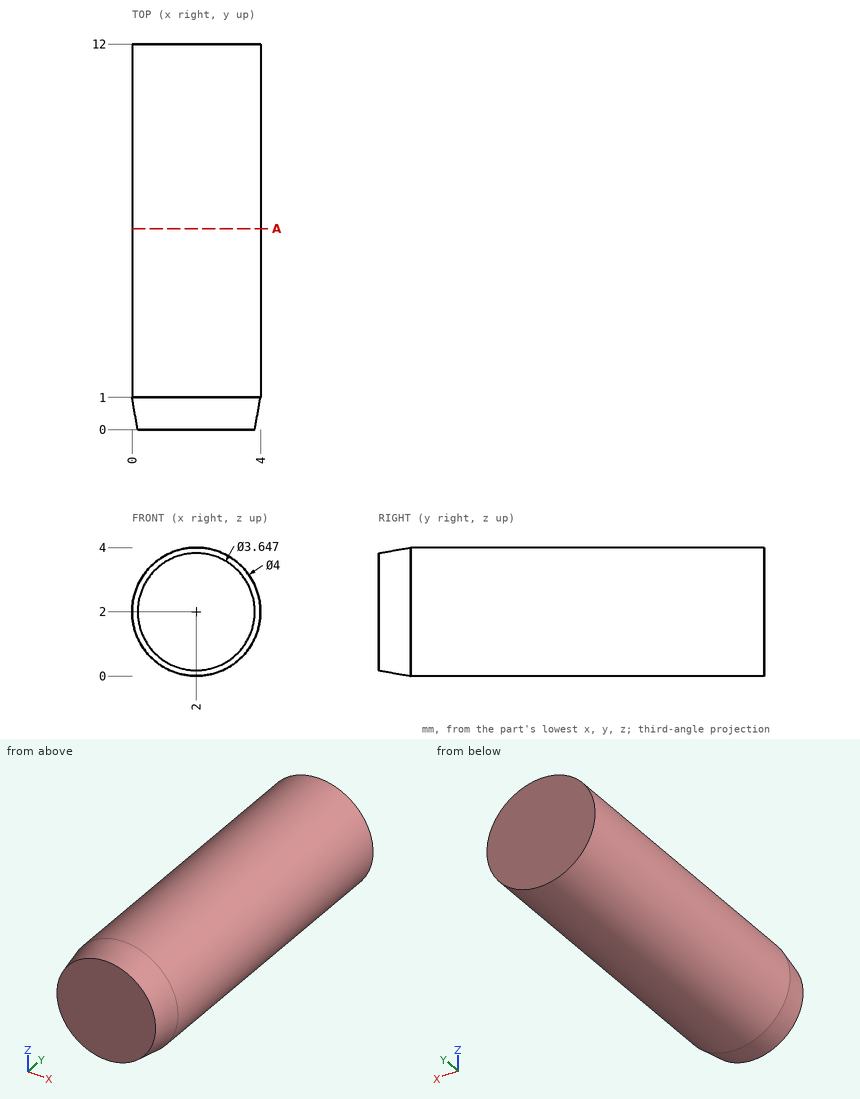
Check sheet for the drawn part. Datum: minimum x, y, z corner. Units: mm. Round coordinates to 2 decimals unless told otherwise and drop trailing zeros. Order: outer loops, then holes, each group sorted by start corner. A loop starts at its lowest first (then second) coordinate and runs counter-clockwise, first axis right, second up.
(1) Go/stop test with a flat-tipped pin: P1, Ø2, axis at x = 1.5, y = 8.5, coming from the -Z side. Record where the tip stops, or that it passes through.
(2) Scan lines: probe 1 along Z at (x, y) = (2.1, 2); probe 2 along Z at (x, y) = (2.9, 4.25) (1 decimal); probe 3 along X at (y, z) = (2, 0.8). Record each from-to range of solid material in increasing order.
(3) Cross-section at A-A, the plane y = 6.25. Enter the section's corners in (x, z).
Check sheet entries:
1. P1: stops at z = 0
2. probe 1: z = 0 to 4
2. probe 2: z = 0.2 to 3.8
2. probe 3: x = 0.4 to 3.6
3. outline: circle Ø4 at (2, 2)
